Geometry: final body of the model. Coordinates: model frame, mm. A direction names the side the tool comes from. Round coordinates to 2 decimals unless told otherwise and drop trailing zeros. Loops run counter-clockwise (first coordinate to the right, second up) from the corner with the lowest first, then second, coordinate; pieces in that order, holes last. Notation, with made-up numbers: (-38.5, 70.5) - (-17.5, 70.5) arc R26 ccw to (-17.5, 103.5) - close; hole circle Ø1 at (-26.75, 67). An arc over 180 degrees is marked (long way). Return JSON: item names as keys, results as strings. Group by question number.
1. Section B-B on z = -15. Return loops of the section in (x, y), and give its area (3 significant figures).
2. Set-up query: faces 1 (the face through (7.3, 3.8, -19.1)), 2 (the face through (7, 4, -12)), 3 (the face through (7.8, 3, -16)), 4 (the face through (3, 4, -11.8)). Return all of +Z, -Z, +X, -X, +Y, -Y with unobstructed straight access to the full face (end or side cutting, diameter ignored); none if empty.
3. Section C-C on y = -4.5. Return loops of the section in (x, z), and give its area (3 significant figures).
4. Material intervals for probe 1 along Z at (x, y) = (6.5, 6.5); probe 2 along X at (y, z) = (3.5, -18.5); probe 3 along Y at (x, z) = (10.5, -5.75), sorted ascending.
5. Section D-D on z = -2.25. Return loops of the section in (x, y).
6. First-contact query: pin 1 Ø2 at (x, z) = (7, -11) entering from -Y; pin 2 Ø4 at (x, z) = (17, -9) entering from +Y; pin 3 Ø4.5 at (y, z) = (4.5, -15) entering from +X. Flat tips, straight axial feed; report the tip coordinate or a pass-through.
7. Section A-A on x = 4. Return loops of the section in (y, z), and give its area (3 significant figures).
from build123d import *

# Parameters (mm, degrees)
BOSS_EXTRUDE1_DEPTH = 19.6
BOSS_EXTRUDE4_DEPTH = 7.8
CHAMFER3_SIZE       = 1


with BuildPart() as part:
    # Sketch1 → Boss-Extrude1 (new body)
    with BuildSketch(Plane.XY):
        Polygon((0, 0), (0, -19.5), (19.5, 0), align=None)
    extrude(amount=-BOSS_EXTRUDE1_DEPTH)

    # Sketch2 → Boss-Extrude4 (add)
    with BuildSketch(Plane(origin=(0, 0, 0), x_dir=(1, 0, 0), z_dir=(0, 1, 0))):
        Polygon((7.8, 19.6), (0, 19.6), (0, 13.7), (0, 11.8), (7.8, 11.8), align=None)
    extrude(amount=BOSS_EXTRUDE4_DEPTH)

    # Chamfer3
    chamfer3_edges = [part.edges().sort_by_distance(p)[0] for p in [
        (7.8, 3.9, -11.8),
        (7.8, 3.9, -19.6),
        (7.8, 7.8, -15.7),
    ]]
    chamfer(chamfer3_edges, length=CHAMFER3_SIZE)


solid = part.part
Taken from the geometry:
{
 "1": {"outline": "(0, -19.5) - (19.5, 0) - (7.8, 0) - (7.8, 6.8) - (6.8, 7.8) - (0, 7.8) - close", "area": "250 mm2"},
 "2": {"face 1": "-Z, +X, +Y", "face 2": "+Z, +X, +Y", "face 3": "+Z, -Z, +X, +Y", "face 4": "+Z, +X, -X, +Y"},
 "3": {"outline": "(0, -19.6) - (15, -19.6) - (15, 0) - (0, 0) - close", "area": "294 mm2"},
 "4": {"probe 1": "-19.6 to -11.8", "probe 2": "0 to 7.8", "probe 3": "-9 to 0"},
 "5": {"outline": "(0, -19.5) - (19.5, 0) - (0, 0) - close"},
 "6": {"pin 1": "y = -13.5", "pin 2": "y = 0", "pin 3": "x = 7.8"},
 "7": {"outline": "(-15.5, -19.6) - (7.8, -19.6) - (7.8, -11.8) - (0, -11.8) - (0, 0) - (-15.5, 0) - close", "area": "365 mm2"}
}
